The listing builds one solid part. Answer for the finished solid, in the listing's coordinates (mm). Coordinates: 2 decimals unless noted, no trailing zeros. Write each loop counter-clockwise with the first axis right and the second up, starting at its lowest first coordinate (ties: lowest second). Pieces come first, ordered by that corner, then holes. Notation, with made-up numbers: M -12,12 L 1,12 A30 cw 1,37 Z; hole C 73,10.5 d7. An arc over 180 degrees is marked long. Answer as CSV lines item,"result".
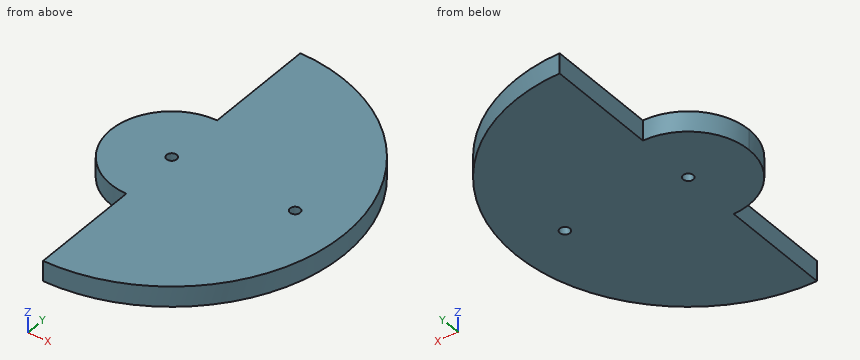
```python
from build123d import *

# Parameters (mm, degrees)
SKETCH_1_R          = 85
EXTRUDE_1_DEPTH     = 10
SKETCH_2_R          = 2.5
CUT_EXTRUDE_1_DEPTH = 121.623380818
SKETCH_3_R          = 2.5
CUT_EXTRUDE_2_DEPTH = 121.623380818
CUT_EXTRUDE_3_DEPTH = 121.623380818
EXTRUDE_START       = -10
SKETCH_5_R          = 2.5
EXTRUDE_2_DEPTH     = 10


with BuildPart() as part:
    # 草图1 → 凸台-拉伸1 (new body)
    with BuildSketch(Plane.XY):
        Circle(SKETCH_1_R)
    extrude(amount=EXTRUDE_1_DEPTH)

    # 草图2 → 切除-拉伸1 (cut, through all)
    with BuildSketch(Plane.XY.offset(10)):
        Circle(SKETCH_2_R)
        with Locations((80, 0)):
            Circle(SKETCH_2_R)
    extrude(amount=-CUT_EXTRUDE_1_DEPTH, mode=Mode.SUBTRACT)

    # 草图3 → 切除-拉伸2 (cut, through all)
    with BuildSketch(Plane(origin=(0, 0, 0), x_dir=(-1, 0, 0), z_dir=(0, 0, -1))):
        with Locations((-60.025485081, 1.009333311)):
            Circle(SKETCH_3_R)
    extrude(amount=-CUT_EXTRUDE_2_DEPTH, mode=Mode.SUBTRACT)

    # 草图4 → 切除-拉伸3 (cut, through all)
    with BuildSketch(Plane(origin=(0, 0, 0), x_dir=(-1, 0, 0), z_dir=(0, 0, -1))):
        with BuildLine():
            ThreePointArc((85, 0), (60.104076401, 60.104076401), (0, 85))
            Line((0, 85), (0, 30))
            ThreePointArc((0, 30), (21.213203436, 21.213203436), (30, 0))
            ThreePointArc((30, 0), (21.213203436, -21.213203436), (0, -30))
            Line((0, -30), (0, -85))
            ThreePointArc((0, -85), (60.104076401, -60.104076401), (85, 0))
        make_face()
    extrude(amount=-CUT_EXTRUDE_3_DEPTH, mode=Mode.SUBTRACT)

    # 草图5 → 凸台-拉伸2 (add)
    with BuildSketch(Plane(origin=(0, 0, 0), x_dir=(-1, 0, 0), z_dir=(0, 0, -1)).offset(EXTRUDE_START)):
        with Locations((-80, 0)):
            Circle(SKETCH_5_R)
    extrude(amount=EXTRUDE_2_DEPTH)


solid = part.part
```
Q1. Straight lines are drawn through the part: line 1 (Y direction, x = 60, z = 7.75); line 2 (X direction, y = -57, z = 7.5); line 3 (X direction, y = 20, z = 2.5). For each, find the intervals that lie inside material, in ascending order.
Output:
line 1,"-60.21 to -1.49, 3.51 to 60.21"
line 2,"0 to 63.06"
line 3,"-22.36 to 82.61"
Q2. Find section C-C (y = -49). Give the vertices of the cut face in (x, z), and give its area (3 significant figures).
Output:
outline,"M 0,0 L 69.46,0 L 69.46,10 L 0,10 Z"
area,"695 mm2"
Q3. Find section A-A (z = 1.75). Give the vertices of the cut face in (x, y).
Output:
outline,"M 0,-85 A85 ccw 0,85 L 0,30 A30 ccw 0,-30 Z; hole C 0,0 d5; hole C 60.03,1.01 d5"
Q4. Find section B-B (x = 77). Give the vertices of the cut face in (y, z), and give its area (3 significant figures).
Output:
outline,"M -36,0 L 36,0 L 36,10 L -36,10 Z"
area,"720 mm2"
Q5. Flat-ended cylindrical pins translate along their axes: pin 1 Ø3 at (x, y) = (0, 0) entering from -Z; pin 2 Ø1.5 at (y, z) = (53, 1.5) entering from +X; pin 3 Ø5 at (y, z) = (47.5, 3.5) entering from -X; pin 4 Ø2 at (x, z) = (39.5, 2) entering from +Y. Find the tip coordinate at first contact, or state that the pin passes through.
Output:
pin 1,"through"
pin 2,"x = 67.04"
pin 3,"x = 0"
pin 4,"y = 75.78"
